Can you work these out from the model? Positions are in its coordinate system, mm. A direction names the side the tool comes from. Round coordinates to 2 decimals unless told otherwise and drop trailing zeros. Loops run counter-clockwise (first coordinate to the right, second up) from the corner with the lowest first, then second, coordinate; pieces in that order, holes last. Notation, with made-up numbers: (83.25, 51.25) -> (137.25, 51.25) arc R15 ccw to (137.25, 58.25) -> close; hole circle Ø1 at (67, 36.25). An arc over 180 degrees is marked (long way). Use a Markdown table: item, result.
from build123d import *

# Parameters (mm, degrees)
SKETCH1_R           = 3.175
BOSS_EXTRUDE1_DEPTH = 6.35
CHAMFER1_START      = 34.302216058
CHAMFER1_OUTLINE_W  = 19.05
CHAMFER1_OUTLINE_H  = 6.35
CHAMFER1_DEPTH      = 8.674261314
FILLET1_R           = 7.62


with BuildPart() as part:
    # Sketch1 → Boss-Extrude1 (new body)
    with BuildSketch(Plane.XY):
        with BuildLine():
            Line((-6.35, 0), (-6.35, 95.25))
            Line((-6.35, 95.25), (-12.7, 95.25))
            ThreePointArc((-12.7, 95.25), (-19.05, 101.6), (-12.7, 107.95))
            Line((-12.7, 107.95), (0, 107.95))
            ThreePointArc((0, 107.95), (4.490128061, 106.090128061), (6.35, 101.6))
            Line((6.35, 101.6), (6.35, 0))
            ThreePointArc((6.35, 0), (0, -6.35), (-6.35, 0))
        make_face()
        Circle(SKETCH1_R, mode=Mode.SUBTRACT)
        with Locations((-12.7, 101.6)):
            Circle(SKETCH1_R, mode=Mode.SUBTRACT)
    extrude(amount=BOSS_EXTRUDE1_DEPTH)

    # Chamfer1: read off the stored shape, not the designer's step
    # Chamfer1 outline → Chamfer1 (add)
    with BuildSketch(Plane(origin=(0, 0, 0), x_dir=(0.49999999999999195, -0.8660254037844434, 0), z_dir=(0.8660254037844433, 0.4999999999999921, 0)).offset(CHAMFER1_START)):
        with Locations((-81.638181024, -3.175)):
            Rectangle(CHAMFER1_OUTLINE_W, CHAMFER1_OUTLINE_H)
    extrude(amount=CHAMFER1_DEPTH)

    # Fillet1
    fillet1_edges = [part.edges().sort_by_distance(p)[0] for p in [
        (-6.35, 79.602954743, 3.175),
        (-15.875, 96.100738686, 3.175),
    ]]
    fillet(fillet1_edges, radius=FILLET1_R)


solid = part.part
1. I want a section at A-A (z = 3). Please give me the cut outline in (x, y) (3 decimals).
Answer sheet:
| item | result |
|---|---|
| outline | (-16.773, 96.729) arc R7.62 cw to (-15.062, 94.693) -> (-7.371, 81.371) arc R7.62 cw to (-6.35, 77.561) -> (-6.35, 0) arc R6.35 ccw to (6.35, 0) -> (6.35, 101.6) arc R6.35 ccw to (0, 107.95) -> (-12.7, 107.95) arc R6.35 ccw to start; hole circle Ø6.35 at (-12.7, 101.6); hole circle Ø6.35 at (0, 0) |
2. I want a section at C-C (y = 76.5). Please give me the cut outline in (x, z), plus the area to 3 significant figures.
Answer sheet:
| item | result |
|---|---|
| outline | (-6.35, 0) -> (6.35, 0) -> (6.35, 6.35) -> (-6.35, 6.35) -> close |
| area | 80.6 mm² |
3. Which directions (+Z, -Z, +X, -X, +Y, -Y) give clear straight access to the entire face, cutting with the end or side of a thin tool? Please do faces 1 (the flat face through (-6.35, 38, 3)), 2 (the flat face through (6.35, 52, 3)).
Answer sheet:
| item | result |
|---|---|
| face 1 | +Z, -Z, -X, -Y |
| face 2 | +Z, -Z, +X, +Y, -Y |
4. Will these pins go through, and if not, where does the flat tip stop? pin 1 Ø5 at (x, y) = (0, 0) entering from +Z; pin 2 Ø1 at (y, z) = (49, 3.5) entering from -X; pin 3 Ø2 at (y, z) = (88.5, 2.5) entering from -X.
Answer sheet:
| item | result |
|---|---|
| pin 1 | passes through |
| pin 2 | stops at x = -6.35 |
| pin 3 | stops at x = -12.06 |
5. I need wall thicknesses on line 1 (Y direction, x = 0, z = 2.75) (3 decimals); line 2 (Y direction, x = -13.25, z = 3.5); line 3 (X direction, y = 62.5, z = 1.5). Which ranges of each line are inside material? Lowest first, please.
Answer sheet:
| item | result |
|---|---|
| line 1 | y = -6.35 to -3.175, 3.175 to 107.95 |
| line 2 | y = 91.55 to 98.47, 104.73 to 107.93 |
| line 3 | x = -6.35 to 6.35 |
6. If we mould it in two halves opening along Y, with no side actions, what happens to faces 3 (the cylindrical face through (-10.993, 104.277, 3.131)), 4 (the cylindrical face through (-0.69, -3.1, 3.13)), 5 (the flat face through (-1, 52, 0)), 6 (the cylindrical face through (-6.617, 79.56, 3.131))? For each: +Y half, -Y half, draft (parallel to the pull), parting line (faces both ways), or undercut.
Answer sheet:
| item | result |
|---|---|
| face 3 | undercut |
| face 4 | undercut |
| face 5 | draft |
| face 6 | -Y half |
7. I want a section at B-B (x = 2). Please give me the cut outline in (y, z), plus the area to 3 significant figures.
Answer sheet:
| item | result |
|---|---|
| outline | (-6.03, 0) -> (-2.47, 0) -> (-2.47, 6.35) -> (-6.03, 6.35) -> close; (2.47, 0) -> (107.63, 0) -> (107.63, 6.35) -> (2.47, 6.35) -> close |
| area | 690 mm² |
